Work out the finished part from the listing and answer in its coordinate system (mm). Face numbers are marked on the shaded views. A direction names the side the tool comes from. Round coordinates to 2 decimals unless told otherwise and drop trailing zeros. Write each loop counter-clockwise with the first axis right and the second up, starting at its lowest first coordinate (ties: lowest second). Pieces come first, ordered by that corner, then holes. Notation, with made-up numbers: (-14.75, 62.25) - (37.25, 62.25) arc R19 ccw to (37.25, 92.25) - close; hole circle Ø7 at (63, 3). An arc over 180 degrees is marked (long way). Write item = value, one per line. Start each with the question number.
from build123d import *

# Parameters (mm, degrees)
SKETCH1_R           = 0.889
SKETCH1_R_2         = 1.875
BOSS_EXTRUDE1_DEPTH = 8
SKETCH2_R           = 4
CUT_EXTRUDE1_DEPTH  = 5.5


with BuildPart() as part:
    # Sketch1 → Boss-Extrude1 (new body)
    with BuildSketch(Plane(origin=(0, 0, 0), x_dir=(1, 0, 0), z_dir=(0, 1, 0))):
        with BuildLine():
            Line((-22.225, 2.5), (-22.225, -2.5))
            Line((-22.225, -2.5), (-7.071067812, -2.5))
            ThreePointArc((-7.071067812, -2.5), (0, -7.5), (7.071067812, -2.5))
            Line((7.071067812, -2.5), (22.225, -2.5))
            Line((22.225, -2.5), (22.225, 2.5))
            Line((22.225, 2.5), (7.071067812, 2.5))
            ThreePointArc((7.071067812, 2.5), (0, 7.5), (-7.071067812, 2.5))
            Line((-7.071067812, 2.5), (-22.225, 2.5))
        make_face()
        with Locations(Location((-19.05, 0, 0), (0, 0, 270))):
            Circle(SKETCH1_R, mode=Mode.SUBTRACT)
        with Locations(Location((0, 0, 0), (0, 0, 270))):
            Circle(SKETCH1_R_2, mode=Mode.SUBTRACT)
        with Locations(Location((19.05, 0, 0), (0, 0, 90))):
            Circle(SKETCH1_R, mode=Mode.SUBTRACT)
    extrude(amount=BOSS_EXTRUDE1_DEPTH)

    # Sketch2 → Cut-Extrude1 (cut)
    with BuildSketch(Plane(origin=(0, 8, 0), x_dir=(1, 0, 0), z_dir=(0, 1, 0))):
        with Locations(Location((0, 0, 0), (0, 0, 270))):
            Circle(SKETCH2_R)
    extrude(amount=-CUT_EXTRUDE1_DEPTH, mode=Mode.SUBTRACT)


solid = part.part
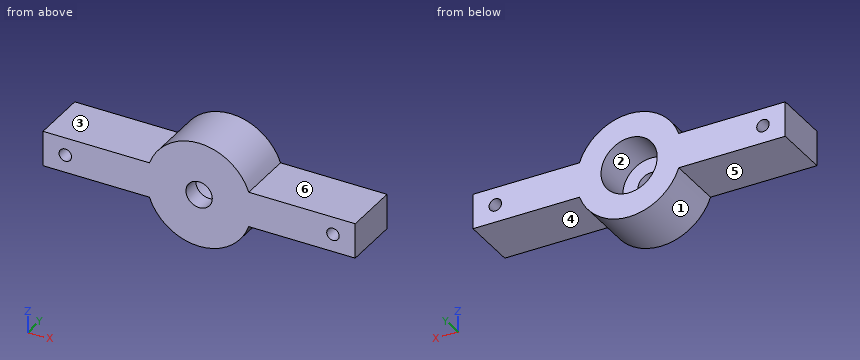
1. Find section D-D on x = -3. Give the vertices of the cut face in (y, z).
2. Find section A-A on x = -19.05. Give the vertices of the cut face in (y, z), plus the area to 3 significant figures.
3. Each of these flat-tipped pins is pushed along its axis until it touches: pin 1 (4 mm diameter, centred on x = 15, y = 4, fed in from +Z); pin 2 (2.5 mm diameter, centred on x = 1, z = 0, fed in from +Y); pin 3 (2.5 mm diameter, centred on x = 16.5, y = 2.5, fed in from -Z). Where does it stop, or does it pass through?
4. Find section C-C on z = -0.5. Give the vertices of the cut face in (x, y) (3 decimals), plus the area to 3 significant figures.
5. Consider line 1 (X direction, y = 5.7, z = 0) (3 decimals); line 2 (X direction, y = 0.8, z = 0) (3 decimals); line 3 (Z direction, x = 19.05, y = 1.5). Determine where each line is inside the solid, lowest interval first.
6. Find section B-B on y = 3.25. Give the vertices of the cut face in (x, z) (3 decimals), plus the area to 3 significant figures.
7. For a pull along X with two mould halves and no side action, classify the marked faces 1, 2 and 3 as released by +X, released by -X, zero draft, split by the parting line, or undercut.
8. Which of the six approach directions +Z, -Z, +X, -X, +Y, -Y give full straight-line access (tool end or side, diameter ignored) to the marked faces 4, 5 and 6?
Answer key:
q1.outline = (0, -6.87) - (8, -6.87) - (8, -2.65) - (2.5, -2.65) - (2.5, 2.65) - (8, 2.65) - (8, 6.87) - (0, 6.87) - close
q2.outline = (0, -2.5) - (8, -2.5) - (8, -0.89) - (0, -0.89) - close; (0, 0.89) - (8, 0.89) - (8, 2.5) - (0, 2.5) - close
q2.area = 25.8 mm²
q3.pin_1 = 2.5
q3.pin_2 = 2.5
q3.pin_3 = -2.5
q4.outline = (-22.225, 0) - (-19.785, 0) - (-19.785, 8) - (-22.225, 8) - close; (-18.315, 0) - (-1.807, 0) - (-1.807, 2.5) - (-3.969, 2.5) - (-3.969, 8) - (-18.315, 8) - close; (1.807, 0) - (18.315, 0) - (18.315, 8) - (3.969, 8) - (3.969, 2.5) - (1.807, 2.5) - close; (19.785, 0) - (22.225, 0) - (22.225, 8) - (19.785, 8) - close
q4.area = 279 mm²
q5.line_1 = -22.225 to -19.939, -18.161 to -4, 4 to 18.161, 19.939 to 22.225
q5.line_2 = -22.225 to -19.939, -18.161 to -1.875, 1.875 to 18.161, 19.939 to 22.225
q5.line_3 = -2.5 to -0.89, 0.89 to 2.5
q6.outline = (-22.225, -2.5) - (-7.071, -2.5) arc R7.5 ccw to (7.071, -2.5) - (22.225, -2.5) - (22.225, 2.5) - (7.071, 2.5) arc R7.5 ccw to (-7.071, 2.5) - (-22.225, 2.5) - close; hole circle Ø1.778 at (-19.05, 0); hole circle Ø8 at (0, 0); hole circle Ø1.778 at (19.05, 0)
q6.area = 270 mm²
q7.face_1 = split by the parting line
q7.face_2 = undercut
q7.face_3 = zero draft
q8.face_4 = -Z, +X, +Y, -Y
q8.face_5 = -Z, -X, +Y, -Y
q8.face_6 = +Z, +X, +Y, -Y
